Here's how the part is built. I have some questions about the finished solid (model axes, mm). Face numbers are marked on the shaded views. A direction names the side the tool comes from. Round coordinates to 2 decimals unless told otherwise and drop trailing zeros. Loops run counter-clockwise (first coordinate to the right, second up) from the corner with the lowest first, then second, coordinate; pieces in that order, holes last. Notation, with made-up numbers: M 48,67 L 89,67 A16 cw 89,93 Z; hole C 2.25,-13 d8. An arc over 180 degrees is marked long. Answer as CSV lines item,"result".
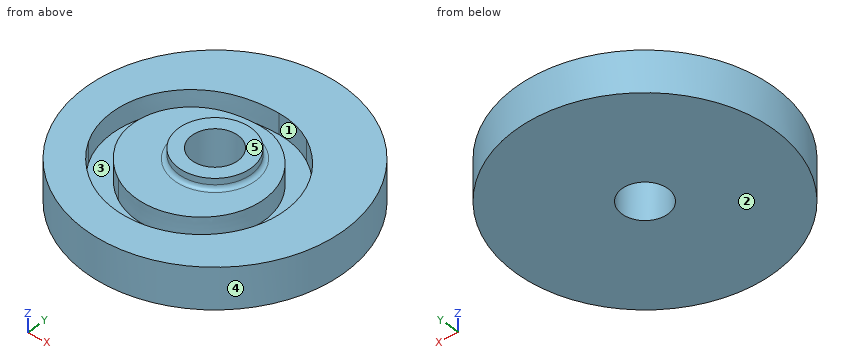
```python
from build123d import *

# Parameters (mm, degrees)
SKETCH_1_R          = 62.5
SKETCH_1_R_2        = 17.5
EXTRUDE_1_DEPTH     = 20
SKETCH_1_3_R        = 17.5
SKETCH_1_3_R_2      = 11.1
EXTRUDE_2_DEPTH     = 25
FILLET_1_R          = 2
CUT_EXTRUDE_3_DEPTH = 10


with BuildPart() as part:
    # 草圖1 → 伸長1 (new body)
    with BuildSketch(Plane.XY):
        Circle(SKETCH_1_R)
        Circle(SKETCH_1_R_2, mode=Mode.SUBTRACT)
    extrude(amount=EXTRUDE_1_DEPTH)

    # 草圖1<3> → 伸長2 (add)
    with BuildSketch(Plane.XY):
        Circle(SKETCH_1_3_R)
        Circle(SKETCH_1_3_R_2, mode=Mode.SUBTRACT)
    extrude(amount=EXTRUDE_2_DEPTH)

    # 圓角1
    fillet_1_edges = [part.edges().sort_by_distance(p)[0] for p in [
        (-17.5, 0, 20),
    ]]
    fillet(fillet_1_edges, radius=FILLET_1_R)

    # 草圖2 → 伸長3 (cut)
    # profile 1 of 2: a face of its own
    with BuildSketch(Plane.XY.offset(20)):
        with BuildLine():
            add(Edge.make_bspline(
                [(-40.703193978, -23.5), (-41.633468538, -21.888717197), (-43.261081238, -18.515622169), (-45.47602304, -11.436735837), (-46.243691745, -2.107968515), (-43.902529687, 8.897505781), (-38.463548338, 18.728740964), (-30.481363737, 26.558580127), (-20.761184619, 31.841785399), (-12.098446566, 34.077729261), (-5.163063209, 34.881869437), (-1.724610104, 35), (0, 35)],
                knots=[0, 0, 0, 0, 0.0625, 0.125, 0.25, 0.375, 0.5, 0.625, 0.75, 0.875, 0.9375, 1, 1, 1, 1], degree=3))
            ThreePointArc((0, 35), (9.058666579, 33.80740392), (17.5, 30.310889132))
            add(Edge.make_bspline(
                [(17.5, 30.310889132), (19.823071752, 28.969663031), (24.242241599, 25.860788384), (31.767486538, 18.159304931), (36.957936485, 8.442419858), (39.023468486, -2.347510431), (38.872672018, -10.560155104), (37.094152942, -18.593345142), (33.679815381, -26.106950798), (28.861351557, -32.744129421), (20.777254706, -40.190094393), (10.741659927, -44.903538266), (-0.034110412, -46.584563974), (-8.185130119, -46.241615161), (-14.797664919, -44.661390317), (-19.864008497, -42.647893398), (-22.312751805, -41.388652043), (-23.5, -40.703193978)],
                knots=[0, 0, 0, 0, 0.0625, 0.125, 0.25, 0.3125, 0.375, 0.4375, 0.5, 0.5625, 0.625, 0.75, 0.8125, 0.875, 0.9375, 0.96875, 1, 1, 1, 1], degree=3))
            ThreePointArc((-23.5, -40.703193978), (-33.234018716, -33.234018716), (-40.703193978, -23.5))
        make_face()
        with BuildLine():
            ThreePointArc((-36.373066959, -21), (-29.69848481, -29.69848481), (-21, -36.373066959))
            add(Edge.make_bspline(
                [(15, 25.980762114), (19.626342308, 23.309742136), (27.962941081, 15.94725242), (35.002577573, -0.237057072), (33.123865827, -19.358084353), (20.586920622, -35.934246999), (-0.118084402, -43.440012631), (-14.591726515, -40.07288538), (-21, -36.373066959)],
                knots=[0, 0, 0, 0, 0.139447987, 0.287926298, 0.449747773, 0.62466703, 0.809633221, 1, 1, 1, 1], degree=3))
            ThreePointArc((15, 25.980762114), (7.764571353, 28.977774789), (0, 30))
            add(Edge.make_bspline(
                [(-36.373066959, -21), (-38.826726203, -16.750137525), (-41.728361124, -7.389186422), (-39.760869449, 6.972263731), (-32.441668175, 18.614971808), (-22.070852951, 26.028055814), (-10.910814995, 29.43602294), (-3.551275269, 30), (0, 30)],
                knots=[0, 0, 0, 0, 0.188917464, 0.373337047, 0.548988681, 0.712236233, 0.861396552, 1, 1, 1, 1], degree=3))
        make_face(mode=Mode.SUBTRACT)
    # profile 2 of 2: a face of its own
    with BuildSketch(Plane.XY.offset(20)):
        with BuildLine():
            add(Edge.make_bspline(
                [(-36.373066959, -21), (-38.826726203, -16.750137525), (-41.728361124, -7.389186422), (-39.760869449, 6.972263731), (-32.441668175, 18.614971808), (-22.070852951, 26.028055814), (-10.910814995, 29.43602294), (-3.551275269, 30), (0, 30)],
                knots=[0, 0, 0, 0, 0.188917464, 0.373337047, 0.548988681, 0.712236233, 0.861396552, 1, 1, 1, 1], degree=3))
            ThreePointArc((0, 30), (7.764571353, 28.977774789), (15, 25.980762114))
            add(Edge.make_bspline(
                [(15, 25.980762114), (19.626342308, 23.309742136), (27.962941081, 15.94725242), (35.002577573, -0.237057072), (33.123865827, -19.358084353), (20.586920622, -35.934246999), (-0.118084402, -43.440012631), (-14.591726515, -40.07288538), (-21, -36.373066959)],
                knots=[0, 0, 0, 0, 0.139447987, 0.287926298, 0.449747773, 0.62466703, 0.809633221, 1, 1, 1, 1], degree=3))
            ThreePointArc((-21, -36.373066959), (-29.69848481, -29.69848481), (-36.373066959, -21))
        make_face()
        with BuildLine():
            ThreePointArc((-32.04293994, -18.5), (-26.162950904, -26.162950904), (-18.5, -32.04293994))
            add(Edge.make_bspline(
                [(12.5, 21.650635095), (14.30005051, 20.611375448), (17.736546036, 18.19228211), (22.05735975, 13.766251439), (25.469897133, 8.589069076), (27.834895803, 2.837183943), (28.986233619, -3.184904344), (28.876055873, -9.377887783), (27.535742309, -15.415921648), (24.990235447, -21.021768672), (21.332338771, -26.062630488), (16.775819727, -30.259430929), (11.450819301, -33.450705308), (5.550233068, -35.577660612), (-0.603962424, -36.53664799), (-6.792105874, -36.274910535), (-12.848540176, -34.833293242), (-16.692189533, -33.0866798), (-18.5, -32.04293994)],
                knots=[0, 0, 0, 0, 0.0625, 0.125, 0.1875, 0.25, 0.3125, 0.375, 0.4375, 0.5, 0.5625, 0.625, 0.6875, 0.75, 0.8125, 0.875, 0.9375, 1, 1, 1, 1], degree=3))
            ThreePointArc((12.5, 21.650635095), (6.470476128, 24.148145657), (0, 25))
            add(Edge.make_bspline(
                [(-32.04293994, -18.5), (-32.728164967, -17.313155438), (-33.927114764, -14.828407043), (-35.558015667, -9.615244062), (-36.119608205, -2.766575398), (-34.400322061, 5.348624633), (-30.388137801, 12.591820816), (-25.469517856, 17.423005266), (-20.794111606, 20.416968225), (-15.767671789, 22.768018014), (-10.206799727, 24.225660689), (-4.442252157, 24.897281873), (-1.474613785, 25), (0, 25)],
                knots=[0, 0, 0, 0, 0.0625, 0.125, 0.25, 0.375, 0.5, 0.625, 0.6875, 0.75, 0.875, 0.9375, 1, 1, 1, 1], degree=3))
        make_face(mode=Mode.SUBTRACT)
    extrude(amount=-CUT_EXTRUDE_3_DEPTH, mode=Mode.SUBTRACT)


solid = part.part
```
1. I want a section at C-C, the plane y = -54. Please give me the cut outline in (x, z).
Evaluation:
outline,"M -31.47,0 L 31.47,0 L 31.47,20 L -31.47,20 Z"
2. I want a section at A-A, the plane z = 13.25. Count the separate pieces of the cut face and the enclosed holes in it, and give its area (3 significant figures).
Evaluation:
separate pieces,"2"
enclosed holes,"2"
area,"9,590 mm²"
3. Which directions (+Z, -Z, +X, -X, +Y, -Y) give clear straight access to the entire face, cutting with the end or side of a thin tool? Please do the marked faces 1 and 2.
Evaluation:
face 1,"+Z"
face 2,"-Z, +X, -X, +Y, -Y"
4. If I drill on line 1 (X direction, y = -6.5, z = 14.5); line 2 (Z direction, x = 56.5, y = -24.5); line 3 (X direction, y = 27.5, z = 15.5), over which ranges is the centre line in solid material (lowest first)? Write a range as [from, to].
Evaluation:
line 1,"x = [-62.16, -45.73], [-35.71, -9], [9, 28.87], [38.88, 62.16]"
line 2,"z = [0, 20]"
line 3,"x = [-56.12, -28.23], [21.78, 56.12]"
5. We'd pull the mould along X, two halves only. Please class the marked faces 3, 4 and 5: pulls with the +X half, pulls with the -X half, needs draft (parallel to the pull), parting line crosses it, or undercut.
Evaluation:
face 3,"undercut"
face 4,"parting line crosses it"
face 5,"needs draft"
6. For P1, Ø10, axis at y = -15.5, z = 14.5, coming from the +X side; P2, Ø1.5, axis at y = -13.5, z = 3.5, coming from the +X side; P3, Ø12, axis at x = 12, z = 15, coming from the +Y side, each with a flat end and sliding along its axis, tell me the tip position at first contact or that it passes through.
Evaluation:
P1,"stops at x = 61.61"
P2,"stops at x = 61.19"
P3,"stops at y = 62.21"
7. I want a section at B-B, the plane x = 40.5. Please give me the cut outline in (y, z).
Evaluation:
outline,"M -47.6,0 L 47.6,0 L 47.6,20 L -47.6,20 Z"
